from build123d import *

# Parameters (mm, degrees)
BOSS_EXTRUDE1_DEPTH = 4
CUT_EXTRUDE1_REACH  = 155.407


with BuildPart() as part:
    # Sketch1 → Boss-Extrude1 (new body)
    with BuildSketch(Plane.XY):
        with BuildLine():
            Line((5, 106.77078252), (5, 111.77078252))
            Line((5, 111.77078252), (-5, 111.77078252))
            Line((-5, 111.77078252), (-5, 106.77078252))
            ThreePointArc((-5, 106.77078252), (-5.540259913, 105.403610666), (-6.869158879, 104.775066959))
            ThreePointArc((-6.869158879, 104.775066959), (0, -105), (6.869158879, 104.775066959))
            ThreePointArc((6.869158879, 104.775066959), (5.540259913, 105.403610666), (5, 106.77078252))
        make_face()
    extrude(amount=BOSS_EXTRUDE1_DEPTH)

    # Sketch2 → Cut-Extrude1 (cut, up to next)
    with BuildSketch(Plane(origin=(0, 0, 0), x_dir=(-1, 0, 0), z_dir=(0, 0, -1)), mode=Mode.PRIVATE) as cut_extrude1_sk1:
        Polygon((-2.5, -2.5), (-2.5, -37.5), (2.5, -37.5), (2.5, -2.5), (37.5, -2.5), (37.5, 2.5), (2.5, 2.5), (2.5, 37.5), (-2.5, 37.5), (-2.5, 2.5), (-37.5, 2.5), (-37.5, -2.5), align=None)
    cut_extrude1_tool1 = extrude(cut_extrude1_sk1.sketch, amount=-CUT_EXTRUDE1_REACH, mode=Mode.PRIVATE) & part.part
    add(cut_extrude1_tool1.solids().sort_by_distance((0, 0, 0))[0], mode=Mode.SUBTRACT)

    # Sketch3 → CSK for M4 Countersunk Flat Head Screw1 (revolve, cut)
    with BuildSketch(Plane(origin=(0, 106.77078252, 4), x_dir=(0, -1, 0), z_dir=(1, 0, 0))):
        Polygon((0, 0), (0, 4), (2.25, 4), (2.25, 2.45), (4.7, 0), align=None)
    revolve(axis=Axis((0, 106.77078252, 10.35), (0, 0, -1)), mode=Mode.SUBTRACT)


solid = part.part
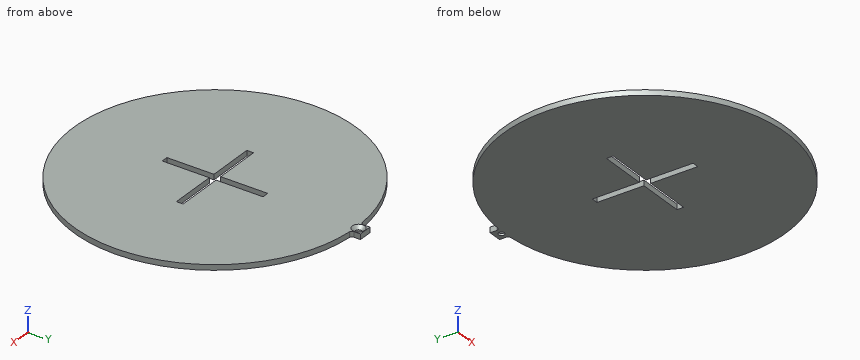
The model under review builds one solid part; all positions refer to its coordinate system, in mm. Round coordinates to 2 decimals unless told otherwise and drop trailing zeros. Order: outer loops, then holes, each group sorted by start corner. A loop starts at its lowest first (then second) coordinate and runs counter-clockwise, first axis right, second up. Notation, with made-up numbers: (-23.75, 51.25) -> (8.25, 51.25) arc R22 cw to (8.25, 79.25) -> close; hole circle Ø10 at (36.25, 14.5). An arc over 180 degrees is marked (long way). Use CSV: the item, a comma, the result in double quotes. Start each with the question number.
(1) Insertion check: pin 1 (1.2 mm diameter, centred on x = 25, z = 2, fed in from +Y); pin 2 (1.2 mm diameter, centred on y = 108.5, z = 1.5, fed in from +X); pin 3 (2.5 mm diameter, centred on x = 0, y = 106.77, fed in from +Z); pin 4 (1.2 mm diameter, centred on x = 16, z = 2.5, fed in from -Y). Each pin has a flat end and moves straight along its axis. Give the tip position at first contact, or say it passes through.
(2) Consider section D-D on x = -63. Write out the cut boundary in (y, z), and give its area (3 significant figures).
(3) Consider section B-B on z = 0.75. Write out the cut boundary in (x, y), and give its area (3 significant figures).
(4) Consider section A-A on y = 0. Write out the cut boundary in (x, z).
(5) Wall thickness on probe 1 along Y at (x, z) = (0, 0.45); probe 2 along Y at (x, z) = (-0.5, 0.5); probe 3 along X at (y, z) = (0, 3.2): over which ranges is each line inside the solid? List them lowest first. Write a range as from..to.
(6) Consider section C-C on x = -25. Write out the cut boundary in (y, z), and give its area (3 significant figures).
Responses:
1,pin 1,"y = 102.13"
1,pin 2,"x = 5"
1,pin 3,"through"
1,pin 4,"y = -103.86"
2,outline,"(-84, 0) -> (84, 0) -> (84, 4) -> (-84, 4) -> close"
2,area,"672 mm²"
3,outline,"(-6.87, 104.78) arc R105 ccw (long way) to (6.87, 104.78) arc R2 cw to (5, 106.77) -> (5, 111.77) -> (-5, 111.77) -> (-5, 106.77) arc R2 cw to start; hole (-37.5, -2.5) -> (-2.5, -2.5) -> (-2.5, -37.5) -> (2.5, -37.5) -> (2.5, -2.5) -> (37.5, -2.5) -> (37.5, 2.5) -> (2.5, 2.5) -> (2.5, 37.5) -> (-2.5, 37.5) -> (-2.5, 2.5) -> (-37.5, 2.5) -> close; hole circle Ø4.5 at (0, 106.77)"
3,area,"34,000 mm²"
4,outline,"(-105, 0) -> (-37.5, 0) -> (-37.5, 4) -> (-105, 4) -> close; (37.5, 0) -> (105, 0) -> (105, 4) -> (37.5, 4) -> close"
5,probe 1,"-105..-37.5, 37.5..104.52, 109.02..111.77"
5,probe 2,"-105..-37.5, 37.5..104.58, 108.96..111.77"
5,probe 3,"-105..-37.5, 37.5..105"
6,outline,"(-101.98, 0) -> (-2.5, 0) -> (-2.5, 4) -> (-101.98, 4) -> close; (2.5, 0) -> (101.98, 0) -> (101.98, 4) -> (2.5, 4) -> close"
6,area,"796 mm²"
